```python
from build123d import *

# Parameters (mm, degrees)
SKETCH2_R           = 13.97
BOSS_EXTRUDE1_DEPTH = 25.4


with BuildPart() as part:
    # Sketch2 → Boss-Extrude1 (new body)
    with BuildSketch(Plane.XY):
        Circle(SKETCH2_R)
        Polygon((-3.666174209, 6.35), (-7.332348419, 0), (-3.666174209, -6.35), (3.666174209, -6.35), (7.332348419, 0), (3.666174209, 6.35), align=None, mode=Mode.SUBTRACT)
    extrude(amount=-BOSS_EXTRUDE1_DEPTH)


solid = part.part
```
Could you check a few things on this model? Use its own coordinates, in mm. A direction names the side the tool comes from. Round coordinates to 2 decimals unless told otherwise and drop trailing zeros. Write each loop counter-clockwise with the first axis right and the second up, starting at its lowest first coordinate (ties: lowest second). Pieces come first, ordered by that corner, then holes.
(1) Suppose I cut it at D-D on x = -10.5. Write out the boundary of the cut face in (y, z), and give its area (3 significant figures).
Findings below:
outline: (-9.21, -25.4) - (9.21, -25.4) - (9.21, 0) - (-9.21, 0) - close
area: 468 mm2
(2) Which directions (+Z, -Z, +X, -X, +Y, -Y) give clear straight access to the entire face, cutting with the end or side of a thin tool? Please do faces 4 (the face through (6, -3, -25.4)), 5 (the face through (0, 6.35, -13)).
Findings below:
face 4: -Z, +X, -X, +Y, -Y
face 5: +Z, -Z
(3) If I drill on probe 1 along Y at (x, z) = (-0.25, -19.75); probe 2 along X at (y, z) = (-2.5, -21.25); probe 3 along Y at (x, z) = (-4, -2.25), over which ranges is the centre line in solid material (lowest first)?
Findings below:
probe 1: y = -13.97 to -6.35, 6.35 to 13.97
probe 2: x = -13.74 to -5.89, 5.89 to 13.74
probe 3: y = -13.39 to -5.77, 5.77 to 13.39
(4) For pin 1 (5 mm diameter, centred on x = -10, z = -12.5, fed in from -Y); pin 2 (1 mm diameter, centred on x = 9.5, y = -2, fed in from +Z); pin 3 (1 mm diameter, centred on x = -7, z = -7.5, fed in from -Y); pin 4 (6 mm diameter, centred on x = -4.5, z = -5, fed in from -Y), each with a flat end and sliding along its axis, tell me the tip position at first contact or that it passes through.
Findings below:
pin 1: stops at y = -11.79
pin 2: stops at z = 0
pin 3: stops at y = -12.37
pin 4: stops at y = -13.89
(5) Thinking about a two-plate mould opening in X: for faces 1 (the face through (0, -6.35, -13)), 2 (the face through (6, -3, 0)), 3 (the face through (-1.82, 13.85, -12.52)), which applies, +X half, -X half, draft (parallel to the pull), parting line (faces both ways), or undercut?
Findings below:
face 1: undercut
face 2: draft
face 3: parting line
(6) Suppose I cut it at A-A on x = 0. Write out the boundary of the cut face in (y, z).
Findings below:
outline: (-13.97, -25.4) - (-6.35, -25.4) - (-6.35, 0) - (-13.97, 0) - close; (6.35, -25.4) - (13.97, -25.4) - (13.97, 0) - (6.35, 0) - close
(7) Suppose I cut it at C-C on y = -5. Write out the boundary of the cut face in (x, z).
Findings below:
outline: (-13.04, -25.4) - (-4.45, -25.4) - (-4.45, 0) - (-13.04, 0) - close; (4.45, -25.4) - (13.04, -25.4) - (13.04, 0) - (4.45, 0) - close
(8) Suppose I cut it at B-B on z = -15.75. Write out the boundary of the cut face in (x, y), and give its area (3 significant figures).
Findings below:
outline: circle Ø27.94 at (0, 0); hole (-7.33, 0) - (-3.67, -6.35) - (3.67, -6.35) - (7.33, 0) - (3.67, 6.35) - (-3.67, 6.35) - close
area: 473 mm2
